Model file for the job. Use its own axes, mm. Face numbers are marked on the shaded views. A direction names the side the tool comes from. Round coordinates to 2 decimals unless told otherwise and drop trailing zeros. Order: outer loops, then holes, each group sorted by start corner. A loop starts at its lowest first (then second) coordinate and runs counter-clockwise, first axis right, second up. Notation, with made-up numbers: (54.25, 30.25) -> (64.25, 30.25) arc R28 cw to (64.25, 56.25) -> close; hole circle Ø6 at (19, 37.5). An arc over 180 degrees is marked (long way). Put each result on its own line as item: value. Start each with the question number.
Q1. Cut at B-B, the plane y = 47.5. List the corners of the cut face in (x, z).
Q2. Pull direction X, two halves, no side cores. Call the marked faces 3, 4 and 5: released by +X, released by -X, zero draft, split by the parting line, or undercut.
Q3. 3-axis set-ups, long thin cutter, end or side, ignore diameter. For the marked faces 1 and 2: which of +Z, -Z, +X, -X, +Y, -Y reach the whole face in a straight line?
Q4. Cut at A-A, the plane x = 0. List the corners of the cut face in (y, z) (3 decimals), and give its area (3 significant figures).
Q5. Cut at D-D, the plane x = 8. List the corners of the cut face in (y, z) (1 decimal), and give its area (3 significant figures).
Q6. Cut at C-C, the plane y = 11. List the corners of the cut face in (x, z).
Q7. Probe L1, parallel to Y at x = -0.5, z = 0.5; L2, parallel to Z at x = -3, y = 39; L3, parallel to Z at x = 11.5, y = 45. List the from-to ranges inside material, lowest first.
Q8. Flat gauge pins, fed straight in: P1, Ø1.5, axis at y = 39, z = -6.5, coming from the -X side; P2, Ø6, axis at y = 18, z = 4, coming from the -X side; P3, Ø12, axis at x = -10, z = -7, coming from the +Y side; P4, Ø1.5, axis at y = 6.5, z = -8, coming from the -X side. Where does each tip first touch, or does it go through?
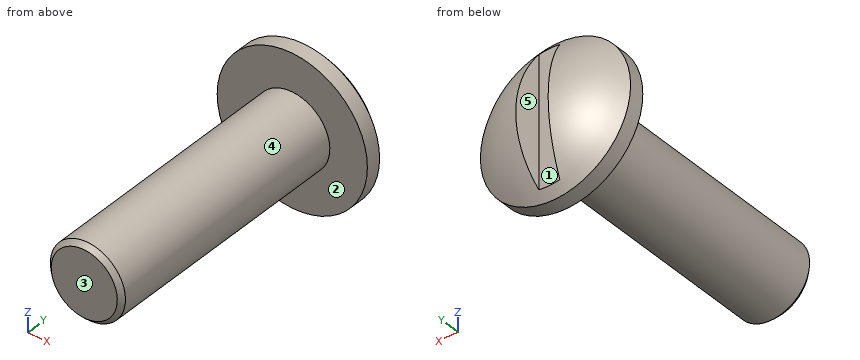
from build123d import *

# Parameters (mm, degrees)
DOME1_FACE_RADIUS       = 12.7
DOME1_HEIGHT            = 5.08
CUT_EXTRUDE2_DEPTH      = 54.881536726
CUT_EXTRUDE2_DEPTH_BACK = 54.881536726
CHAMFER1_SIZE           = 0.762


with BuildPart() as part:
    # Sketch5 → Revolve2 (revolve)
    with BuildSketch(Plane.XY, mode=Mode.PRIVATE) as revolve2_sk:
        Polygon((0, 0), (-6.35, 0), (-6.35, 43.18), (-12.7, 43.18), (-12.7, 45.72), (0, 45.72), (0, 43.18), align=None)
    revolve(revolve2_sk.sketch.rotate(Axis((0, 0, 0), (0, -1, 0)), 270), axis=Axis((0, 0, 0), (0, -1, 0)))

    # Dome1: a dome of height H over a round flat face of radius A is a cap of a sphere of radius (A * A + H * H) / (2 * H)
    dome1_r = (DOME1_FACE_RADIUS * DOME1_FACE_RADIUS + DOME1_HEIGHT * DOME1_HEIGHT) / (2 * DOME1_HEIGHT)
    dome1_base = Plane((0, 45.72, 0), z_dir=(0, 1, 0))
    with Locations(dome1_base.offset(DOME1_HEIGHT - dome1_r)):
        dome1_ball = Sphere(dome1_r, mode=Mode.PRIVATE)
    add(split(dome1_ball, bisect_by=dome1_base, keep=Keep.TOP, mode=Mode.PRIVATE))

    # Sketch7 → Cut-Extrude2 (cut, two sides: drawn at the far end of the back side and taken through both)
    with BuildSketch(Plane.XY.offset(-CUT_EXTRUDE2_DEPTH_BACK)):
        Polygon((-32.713179339, 162.446628615), (-2.742527685, 50.594633903), (-1.776668941, 46.99), (1.776668941, 46.99), (2.742527685, 50.594633903), (32.713179339, 162.446628615), (32.713179339, 394.042040328), (-32.713179339, 394.042040328), align=None)
    extrude(amount=CUT_EXTRUDE2_DEPTH + CUT_EXTRUDE2_DEPTH_BACK, mode=Mode.SUBTRACT)

    # Chamfer1
    chamfer1_edges = [part.edges().sort_by_distance(p)[0] for p in [
        (0, 0, -6.35),
    ]]
    chamfer(chamfer1_edges, length=CHAMFER1_SIZE)


solid = part.part
Ans:
1. outline: (-1.91, -10.34) -> (-1.91, 10.34) arc R10.52 ccw to start; (1.91, -10.34) arc R10.52 ccw to (1.91, 10.34) -> close
2. face 3: zero draft
2. face 4: split by the parting line
2. face 5: undercut
3. face 1: +Z, -Z, +Y
3. face 2: -Y
4. outline: (0, -5.588) -> (0.762, -6.35) -> (43.18, -6.35) -> (43.18, -12.7) -> (45.72, -12.7) arc R18.415 ccw to (46.99, -11.216) -> (46.99, 11.216) arc R18.415 ccw to (45.72, 12.7) -> (43.18, 12.7) -> (43.18, 6.35) -> (0.762, 6.35) -> (0, 5.588) -> close
4. area: 643 mm^2
5. outline: (43.2, -9.9) -> (45.7, -9.9) arc R16.6 ccw to (45.7, 9.9) -> (43.2, 9.9) -> close
5. area: 93.8 mm^2
6. outline: circle Ø12.7 at (0, 0)
7. L1: y = 0 to 46.99
7. L2: z = -5.6 to 5.6
7. L3: z = -5.39 to 5.39
8. P1: stops at x = -2.69
8. P2: stops at x = -6.27
8. P3: stops at y = 49.72
8. P4: passes through
